Could you check a few things on this drawing? It's one solid part, dimensions in mm from its lowest x, y, z. Coordinates: 2 decimals unless noted, no trailing zeros. Order: outer loops, then holes, each group sorted by start corner. A loop starts at its lowest first (then second) coordinate and runs counter-clockwise, first axis right, second up.
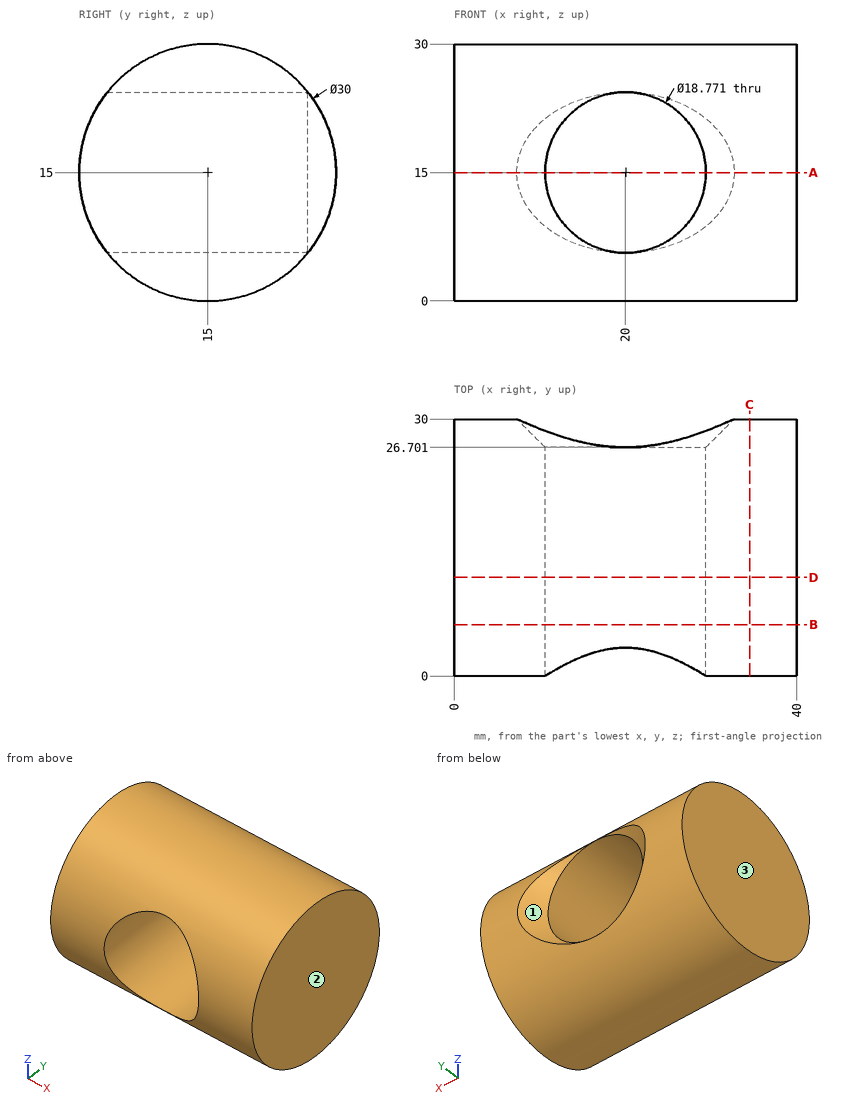
1. Thinking about a two-plate mould opening in X: for the marked faces 1, 2 and 3, which applies, pulls with the +X half, pulls with the -X half, needs draft (parallel to the pull), parting line crosses it, or undercut?
Completed:
face 1: undercut
face 2: pulls with the +X half
face 3: pulls with the -X half
2. I'm going to push flat-ended pins straight in: pin 1 (2 mm diameter, centred on x = 32.5, z = 10, fed in from +Y); pin 2 (10 mm diameter, centred on x = 17.5, z = 8, fed in from +Y); pin 3 (2 mm diameter, centred on x = 19.5, y = 9, fed in from -Z). Where does each tip first touch, or does it pass through?
Completed:
pin 1: stops at y = 29.46
pin 2: stops at y = 27.95
pin 3: stops at z = 0.86
3. Imagine slicing it at D-D on y = 11.5. Please give me the cut outline in (x, z) (1 decimal).
Completed:
outline: (0, 0.4) - (40, 0.4) - (40, 29.6) - (0, 29.6) - close; hole circle Ø18.8 at (20, 15)
4. Imagine slicing it at C-C on x = 34.5. Please give me the cut outline in (y, z), then the cut area to 3 significant figures.
Completed:
outline: circle Ø30 at (15, 15)
area: 707 mm2
5. Imagine slicing it at A-A on z = 15. Please give me the cut outline in (x, y) (1 decimal).
Completed:
outline: (0, 0) - (10.6, 0) - (10.6, 26.7) - (7.3, 30) - (0, 30) - close; (29.4, 0) - (40, 0) - (40, 30) - (32.7, 30) - (29.4, 26.7) - close
6. Imagine slicing it at B-B on y = 6. Please give me the cut outline in (x, z) (1 decimal).
Completed:
outline: (0, 3) - (40, 3) - (40, 27) - (0, 27) - close; hole circle Ø18.8 at (20, 15)
7. Please list where these lines run through material, in increasing order: probe 1 along X at (y, z) = (19, 15) (1 decimal); probe 2 along Y at (x, z) = (36.5, 14.5); probe 3 along Z at (x, y) = (17, 24).
Completed:
probe 1: x = 0 to 10.6, 29.4 to 40
probe 2: y = 0.01 to 29.99
probe 3: z = 3 to 6.11, 23.89 to 27
